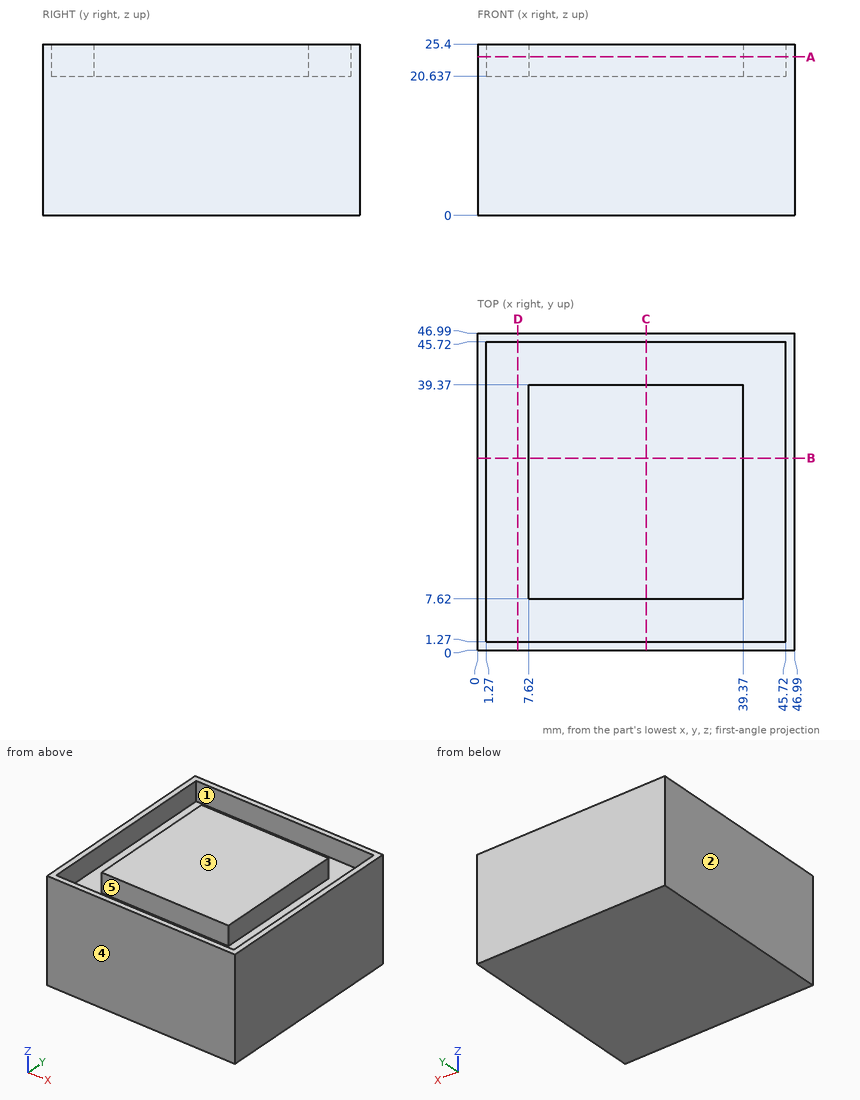
Answer from the drawing. Dimensions are ordinates in mm from the lowest x, y and z of the part. A direction names the side the tool comes from. Give positions to 0.01 mm unless a question says otherwise; leave off trailing zeros. Order: outer loops, then holes, each group sorted by start corner. A loop starts at its lowest first (then second) coordinate and runs counter-clockwise, first axis right, second up.
(1) For the marked faces 4 and 5, determine the directions among +Z, -Z, +X, -X, +Y, -Y from which every point of the face is accessible in a straight line to the end or side of a thin tool.
(2) For a pull along X with two mould halves and no side action, classify the marked faces 1, 2 and 3 as released by +X, released by -X, zero draft, split by the parting line, or undercut.
(3) Straight lines are drawn through the part: L1, parallel to X at y = 43.5, z = 23.5; L2, parallel to X at y = 26.5, z = 22; L3, parallel to Z at x = 6.5, y = 44.5. For each, find the intervals that lie inside material, in ascending order.
(4) Find section D-D (x = 6). Give the vertices of the cut face in (y, z), plus the area to 3 significant figures.
(5) Find section A-A (z = 23.5). Give the vertices of the cut face in (x, y), plus the area to 3 significant figures.
(6) Find section B-B (y = 28.5). Give the vertices of the cut face in (x, z).
Result sheet:
1. face 4: +Z, -Z, +X, -X, -Y
1. face 5: +Z
2. face 1: undercut
2. face 2: released by -X
2. face 3: zero draft
3. L1: x = 0 to 1.27, 45.72 to 46.99
3. L2: x = 0 to 1.27, 7.62 to 39.37, 45.72 to 46.99
3. L3: z = 0 to 20.64
4. outline: (0, 0) - (46.99, 0) - (46.99, 25.4) - (45.72, 25.4) - (45.72, 20.64) - (1.27, 20.64) - (1.27, 25.4) - (0, 25.4) - close
4. area: 982 mm2
5. outline: (0, 0) - (46.99, 0) - (46.99, 46.99) - (0, 46.99) - close; (7.62, 7.62) - (39.37, 7.62) - (39.37, 39.37) - (7.62, 39.37) - close; hole (1.27, 1.27) - (45.72, 1.27) - (45.72, 45.72) - (1.27, 45.72) - close
5. area: 1,240 mm2
6. outline: (0, 0) - (46.99, 0) - (46.99, 25.4) - (45.72, 25.4) - (45.72, 20.64) - (39.37, 20.64) - (39.37, 25.4) - (7.62, 25.4) - (7.62, 20.64) - (1.27, 20.64) - (1.27, 25.4) - (0, 25.4) - close
